from build123d import *

# Parameters (mm, degrees)
SKETCH1_R                      = 46.5
SKETCH1_R_2                    = 38
BOSS_EXTRUDE1_DEPTH            = 3
SKETCH2_R                      = 41
SKETCH2_R_2                    = 38
BOSS_EXTRUDE2_DEPTH            = 100
SKETCH4_W                      = 1.7272
SKETCH4_H                      = 3
F_4_CLEARANCE_HOLE1_AT_2_COUNT = 2
F_4_CLEARANCE_HOLE1_AT_2_PITCH = 59.39696962
F_4_CLEARANCE_HOLE1_AT_3_COUNT = 2
F_4_CLEARANCE_HOLE1_AT_3_PITCH = 84
F_4_CLEARANCE_HOLE1_AT_4_COUNT = 2
F_4_CLEARANCE_HOLE1_AT_4_PITCH = 59.39696962
SKETCH5_R                      = 3.125
CUT_EXTRUDE1_DEPTH             = 3
BOSS_EXTRUDE3_START            = -2
BOSS_EXTRUDE3_DEPTH            = 7
CIRPATTERN3_COUNT              = 4
CUT_EXTRUDE2_DEPTH             = 120.685003238


with BuildPart() as part:
    # Sketch1 → Boss-Extrude1 (new body)
    with BuildSketch(Plane(origin=(0, 0, 0), x_dir=(1, 0, 0), z_dir=(0, 1, 0))):
        with Locations(Location((0, 0, 0), (0, 0, 270))):
            Circle(SKETCH1_R)
        with Locations(Location((0, 0, 0), (0, 0, 270))):
            Circle(SKETCH1_R_2, mode=Mode.SUBTRACT)
    extrude(amount=BOSS_EXTRUDE1_DEPTH)

    # Sketch2 → Boss-Extrude2 (add)
    with BuildSketch(Plane(origin=(0, 3, 0), x_dir=(1, 0, 0), z_dir=(0, 1, 0))):
        with Locations(Location((0, 0, 0), (0, 0, 270))):
            Circle(SKETCH2_R)
        with Locations(Location((0, 0, 0), (0, 0, 270))):
            Circle(SKETCH2_R_2, mode=Mode.SUBTRACT)
    extrude(amount=BOSS_EXTRUDE2_DEPTH)

    # Sketch4 → #4 Clearance Hole1 (revolve, cut)
    with BuildSketch(Plane(origin=(-29.69848481, 3, -29.69848481), x_dir=(0, 0, 1), z_dir=(1, 0, 0))):
        with Locations((0.8636, 1.5)):
            Rectangle(SKETCH4_W, SKETCH4_H)
    f_4_clearance_hole1 = revolve(axis=Axis((-29.69848481, 9.35, -29.69848481), (0, -1, 0)), mode=Mode.SUBTRACT)

    # #4 Clearance Hole1 at 2: #4 Clearance Hole1 ×2
    with Locations(*[(i * F_4_CLEARANCE_HOLE1_AT_2_PITCH, 0, 0) for i in range(1, F_4_CLEARANCE_HOLE1_AT_2_COUNT)]):
        add(f_4_clearance_hole1, mode=Mode.SUBTRACT)

    # #4 Clearance Hole1 at 3: #4 Clearance Hole1 ×2
    with Locations(*[Vector(0.7071067811865476, 0, 0.7071067811865476) * (i * F_4_CLEARANCE_HOLE1_AT_3_PITCH) for i in range(1, F_4_CLEARANCE_HOLE1_AT_3_COUNT)]):
        add(f_4_clearance_hole1, mode=Mode.SUBTRACT)

    # #4 Clearance Hole1 at 4: #4 Clearance Hole1 ×2
    with Locations(*[(0, 0, i * F_4_CLEARANCE_HOLE1_AT_4_PITCH) for i in range(1, F_4_CLEARANCE_HOLE1_AT_4_COUNT)]):
        add(f_4_clearance_hole1, mode=Mode.SUBTRACT)

    # Sketch5 → Cut-Extrude1 (cut)
    with BuildSketch(Plane(origin=(0, 3, 0), x_dir=(1, 0, 0), z_dir=(0, 1, 0))):
        with Locations((-29.69848481, 29.69848481)):
            Circle(SKETCH5_R)
    cut_extrude1 = extrude(amount=CUT_EXTRUDE1_DEPTH, mode=Mode.SUBTRACT)

    # Sketch6 → Boss-Extrude3 (add)
    with BuildSketch(Plane(origin=(0, 3, 0), x_dir=(1, 0, 0), z_dir=(0, 1, 0)).offset(BOSS_EXTRUDE3_START)):
        with BuildLine():
            ThreePointArc((-31.890308819, 25.76835663), (-26.516504294, 26.516504294), (-25.76835663, 31.890308819))
            ThreePointArc((-25.76835663, 31.890308819), (-26.313305576, 31.442168336), (-26.850462289, 30.984716795))
            ThreePointArc((-26.850462289, 30.984716795), (-27.488776119, 27.488776119), (-30.984716795, 26.850462289))
            ThreePointArc((-30.984716795, 26.850462289), (-31.442168336, 26.313305576), (-31.890308819, 25.76835663))
        make_face()
    boss_extrude3 = extrude(amount=BOSS_EXTRUDE3_DEPTH)

    # CirPattern3: Cut-Extrude1, Boss-Extrude3 ×4 about axis
    cirpattern3_axis = Axis((0, 0, 0), (0, 1, 0))
    add([cut_extrude1.rotate(cirpattern3_axis, i * 360 / CIRPATTERN3_COUNT) for i in range(1, CIRPATTERN3_COUNT)], mode=Mode.SUBTRACT)
    add([boss_extrude3.rotate(cirpattern3_axis, i * 360 / CIRPATTERN3_COUNT) for i in range(1, CIRPATTERN3_COUNT)])

    # Sketch7 → Cut-Extrude2 (cut, through all)
    with BuildSketch(Plane(origin=(0, 3, 0), x_dir=(1, 0, 0), z_dir=(0, 1, 0))):
        with BuildLine():
            Line((43, -17.69887002), (43, 17.69887002))
            ThreePointArc((43, 17.69887002), (46.5, 0), (43, -17.69887002))
        make_face()
    extrude(amount=-CUT_EXTRUDE2_DEPTH, mode=Mode.SUBTRACT)


solid = part.part
Check sheet for the modelled part. Datum: model origin and axes. Units: mm. A direction names the side the tool comes from. Round coordinates to 2 decimals unless told otherwise and drop trailing zeros. Loops run counter-clockwise (first coordinate to the right, second up) from the corner with the lowest first, then second, coordinate; pieces in that order, holes last. Notation, with made-up numbers: M 29.25,77 L 83.25,77 A15 cw 83.25,85 Z; hole C 40,2 d1. An arc over 180 degrees is marked long. One line per item, written item: value.
(1) Thickness scan on line 1 (Z direction, x = -1, y = 6); line 2 (X direction, y = 68, z = 0); line 3 (X direction, y = 12, z = 27). Record the ranges inside material, lowest first.
Computed values:
line 1: z = -40.99 to -37.99, 37.99 to 40.99
line 2: x = -41 to -38, 38 to 41
line 3: x = -30.85 to -26.74, 26.74 to 30.85
(2) Sectioned sample at B-B, the plane x = 0. Record the cut outline in (y, z), then the cut area to 3 significant figures.
Computed values:
outline: M 0,-46.5 L 3,-46.5 L 3,-41 L 103,-41 L 103,-38 L 0,-38 Z; M 0,38 L 103,38 L 103,41 L 3,41 L 3,46.5 L 0,46.5 Z
area: 651 mm^2
(3) Sectioned sample at C-C, the plane y = 24. Record the cut outline in (x, z).
Computed values:
outline: C 0,0 d82; hole C 0,0 d76
(4) Release check for a two-part mould opening along Y. For faces 3 (the face through (-28, 6, 28)), 4 (the face through (-26.496, 4.451, 26.537)) record: +Y half, -Y half, draft (parallel to the pull), parting line (faces both ways), or undercut.
Computed values:
face 3: undercut
face 4: draft
(5) Depth check by flat-ended pin: pin 1 Ø2 at (x, z) = (27, 26.5) entering from -Y; pin 2 Ø10 at (y, z) = (33.5, -26) entering from -X; pin 3 Ø1.3 at (x, z) = (29, -29) entering from -Y; pin 4 Ø6 at (x, y) = (-15, 80) entering from +Z. Enter the tip coordinate at first touch or a pass-through.
Computed values:
pin 1: stops at y = 0
pin 2: stops at x = -35.21
pin 3: stops at y = 6
pin 4: stops at z = 39.2
(6) Sectioned sample at A-A, the plane z = 0. Record the cut outline in (x, y).
Computed values:
outline: M -46.5,0 L -38,0 L -38,103 L -41,103 L -41,3 L -46.5,3 Z; M 38,0 L 43,0 L 43,3 L 41,3 L 41,103 L 38,103 Z
(7) Access from +Z, -Z, +X, -X, +Y, -Y to the whole of each face (thin tool, end or side, straight path). Record for faces 1 (the face through (27.53, 4.48, 27.45)), 2 (the face through (29.18, 1.479, 31.346)).
Computed values:
face 1: none
face 2: -Y
